Verification items for the finished model (mm, model axes). Face numbers are marked on the shaded views. Round coordinates to 2 decimals unless told otherwise and drop trailing zeros. Loops run counter-clockwise (first coordinate to the right, second up) from the corner with the lowest first, then second, coordinate; pieces in that order, holes last. Notation, with made-up numbers: (-10, 38.5) - (27, 38.5) arc R18 ccw to (27, 72.5) - close; hole circle Ø8 at (68.5, -40). An arc over 180 degrees is marked (long way). Use a Markdown table: item, result. Add a question column.
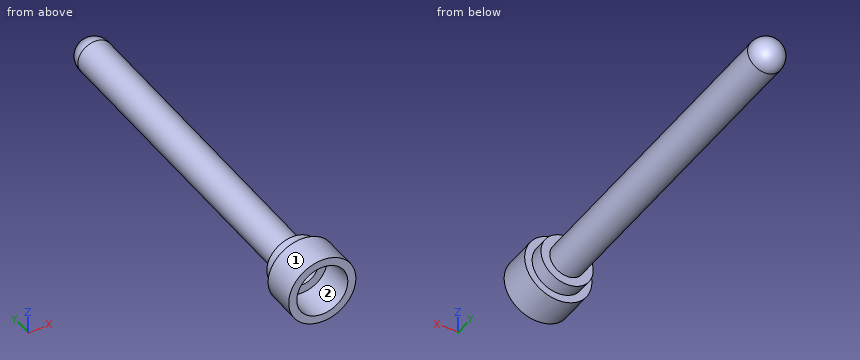
```python
from build123d import *

# Parameters (mm, degrees)
F0_R     = 3.205
F0_R_2   = 2.435
F1_DEPTH = 3.26
F2_R     = 2.491032
F2_R_2   = 1.595
F3_DEPTH = 1.4
F4_R     = 1.651158
F5_DEPTH = 31.52


with BuildPart() as f1:
    # F0 (on Front) → F1 (new body)
    with BuildSketch(Plane.XZ):
        Circle(F0_R)
        Circle(F0_R_2, mode=Mode.SUBTRACT)
    extrude(amount=-F1_DEPTH)

    # F2 (on face) → F3 (join)
    with BuildSketch(Plane(origin=(0, 3.26, 0), x_dir=(-1, 0, 0), z_dir=(0, 1, 0))):
        Circle(F2_R)
        Circle(F2_R_2, mode=Mode.SUBTRACT)
    extrude(amount=F3_DEPTH)

    # F4 (on face) → F5 (join)
    with BuildSketch(Plane(origin=(0, 4.66, 0), x_dir=(-1, 0, 0), z_dir=(0, 1, 0))):
        Circle(F4_R)
    extrude(amount=F5_DEPTH)

    # F7 (on face) → F8 (revolve)
    with BuildSketch(Plane(origin=(0, 36.18, 0), x_dir=(-1, 0, 0), z_dir=(0, 1, 0))):
        with BuildLine():
            Line((0, 1.656466), (0, -1.656466))
            ThreePointArc((0, -1.656466), (1.656466, 0), (0, 1.656466))
        make_face()
    revolve(axis=Axis((0, 36.18, 0), (0, 0, -1)))


solid = f1.part
```
Q1. Section check B-B on z = 0. Record the cut outline in (x, y) (1 decimal), plus the area to 3 significant figures.
Q2. Section check D-D on z = -2. Record the cut outline in (x, y) (3 decimals), plus the area to 3 significant figures.
Q3. Section check A-A on x = 0. Record the cut outline in (y, z) (1 decimal), plus the area to 3 significant figures.
Q4. Release check for a two-part mould opening along X. For the marked faces 1 and 2 record: +X half, -X half, draft (parallel to the pull), parting line (faces both ways), or undercut.
Q5. Go/stop test with flat-tipped pins: pin 1 Ø2.5 at (x, z) = (0, 0) entering from -Y; pin 2 Ø1.5 at (x, y) = (-1.5, 30) entering from +Z; pin 3 Ø1 at (x, z) = (1, 2.5) entering from +Y. Record where each tip stops, or that it passes through.
Q6. Section check C-C on y = 25. Record the cut outline in (x, z), plus the area to 4 significant figures.
Q7. Thickness scan on line 1 along Z through (x, y) = (0, 2) (3 decimals); line 2 along Z through (x, y) = (0, 4) (3 decimals); line 3 along Y through (x, z) = (-0.5, 0). Record the ranges inside material, lowest first.
Determined:
| question | item | result |
|---|---|---|
| 1 | outline | (-3.2, 0) - (-2.4, 0) - (-2.4, 3.3) - (-1.6, 3.3) - (-1.6, 4.7) - (1.6, 4.7) - (1.6, 3.3) - (2.4, 3.3) - (2.4, 0) - (3.2, 0) - (3.2, 3.3) - (2.5, 3.3) - (2.5, 4.7) - (1.7, 4.7) - (1.7, 36) arc R1.7 ccw (long way) to (-1.7, 36) - (-1.7, 4.7) - (-2.5, 4.7) - (-2.5, 3.3) - (-3.2, 3.3) - close |
| 1 | area | 116 mm² |
| 2 | outline | (-2.504, 0) - (-1.389, 0) - (-1.389, 3.26) - (1.389, 3.26) - (1.389, 0) - (2.504, 0) - (2.504, 3.26) - (1.485, 3.26) - (1.485, 4.66) - (-1.485, 4.66) - (-1.485, 3.26) - (-2.504, 3.26) - close |
| 2 | area | 11.4 mm² |
| 3 | outline | (0, -3.2) - (3.3, -3.2) - (3.3, -2.5) - (4.7, -2.5) - (4.7, -1.7) - (36, -1.7) arc R1.7 ccw (long way) to (36, 1.7) - (4.7, 1.7) - (4.7, 2.5) - (3.3, 2.5) - (3.3, 3.2) - (0, 3.2) - (0, 2.4) - (3.3, 2.4) - (3.3, 1.6) - (4.7, 1.6) - (4.7, -1.6) - (3.3, -1.6) - (3.3, -2.4) - (0, -2.4) - close |
| 3 | area | 116 mm² |
| 4 | face 1 | parting line |
| 4 | face 2 | undercut |
| 5 | pin 1 | stops at y = 4.66 |
| 5 | pin 2 | stops at z = 1.47 |
| 5 | pin 3 | stops at y = 4.66 |
| 6 | outline | circle Ø3.3 at (0, 0) |
| 6 | area | 8.565 mm² |
| 7 | line 1 | z = -3.205 to -2.435, 2.435 to 3.205 |
| 7 | line 2 | z = -2.491 to -1.595, 1.595 to 2.491 |
| 7 | line 3 | y = 4.66 to 37.76 |
